For this review, use the dimensioned drawing (mm, ordinates from the lowest corner) and the shaded views. Coordinates: 2 decimals unless noted, no trailing zeros. Loops run counter-clockwise (first coordinate to the right, second up) from the corner with the lowest first, then second, coordinate; pieces in that order, holes last. Notation, with made-up numbers: M 25,16.25 L 31,16.25 A19 ccw 31,41.25 Z; hole C 46,-34 d3. An arc over 180 degrees is marked long. One line per item, written item: value.
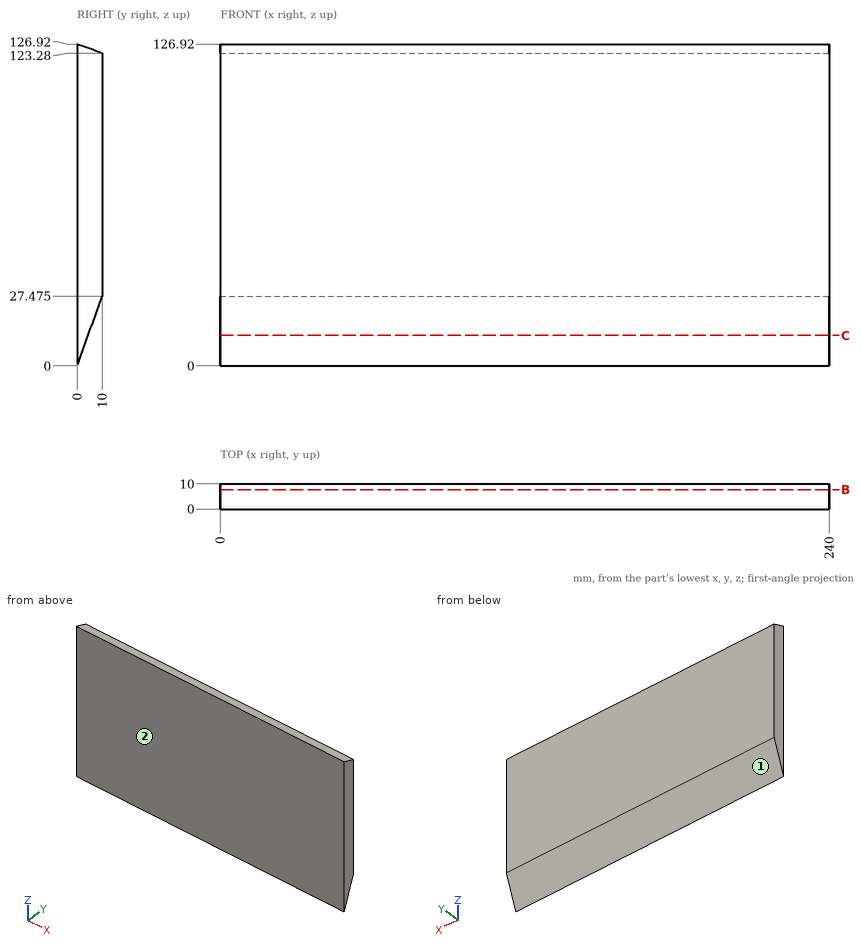
(1) We need section C-C on z = 12. State the section outline as (x, y) points, then the cut area to 3 significant figures.
Reply:
outline: M 0,0 L 240,0 L 240,4.37 L 0,4.37 Z
area: 1,050 mm2
(2) Mouldability with a two-part tool opening along Y and no side actions: class the marked faces 1 and 2 as released by +Y, released by -Y, zero draft, split by the parting line, or undercut.
Reply:
face 1: released by +Y
face 2: released by -Y
(3) To check wall thickness, follow line 1 along Y through (x, z) = (181, 22); line 2 along Y through (x, z) = (15.5, 26.5) (1 decimal). State the ranges of each line that lie inside material, in increasing order. Write a range as [from, to].
Reply:
line 1: y = [0, 8.01]
line 2: y = [0, 9.6]
(4) We need section B-B on y = 7.75. State the section outline as (x, z) points, then the cut area to 3 significant figures.
Reply:
outline: M 0,21.29 L 240,21.29 L 240,124.1 L 0,124.1 Z
area: 24,700 mm2
(5) Insertion check: pin 1 (1.5 mm diameter, centred on x = 176, y = 7, fed in from +Z) (1 decimal). The pin has a flat end and moves straight along its axis. Give the tip position at first contact, or say it passes through.
Reply:
pin 1: stops at z = 124.6
